CAD build for the part. Positions are in the model's coordinates, mm. Face numbers are marked on the shaded views. A direction names the side the tool comes from. Give positions to 0.01 mm unless a question says otherwise; leave off trailing zeros. Write each loop counter-clockwise with the first axis right and the second up, starting at its lowest first coordinate (ties: lowest second). Pieces come first, ordered by that corner, then holes. Notation, with made-up numbers: (62.5, 77.25) - (70.5, 77.25) arc R23 cw to (70.5, 107.25) - close; hole circle Ø6 at (-14, 75.5). An arc over 180 degrees is marked (long way). Answer as a JSON object with one key per item and string values.
from build123d import *

# Parameters (mm, degrees)
SKETCH1_R               = 15.5
SKETCH1_R_2             = 13.5
BOSS_EXTRUDE1_DEPTH     = 18
SKETCH1_3_R             = 13.5
BOSS_EXTRUDE2_DEPTH     = 3
SKETCH2_R               = 1.65
SKETCH2_R_2             = 5.2
CUT_EXTRUDE4_DEPTH      = 41
CUT_EXTRUDE5_DEPTH      = 2
CUT_EXTRUDE6_DEPTH      = 20
CUT_EXTRUDE6_DEPTH_BACK = 16
BOSS_EXTRUDE3_START     = 9
SKETCH5_R               = 15.5
SKETCH5_R_2             = 13.5
BOSS_EXTRUDE3_DEPTH     = 9


with BuildPart() as part:
    # Sketch1 → Boss-Extrude1 (new body)
    with BuildSketch(Plane(origin=(0, 0, 0), x_dir=(1, 0, 0), z_dir=(0, 1, 0))):
        with Locations(Location((0, 0, 0), (0, 0, 270))):
            Circle(SKETCH1_R)
        with Locations(Location((0, 0, 0), (0, 0, 270))):
            Circle(SKETCH1_R_2, mode=Mode.SUBTRACT)
    extrude(amount=BOSS_EXTRUDE1_DEPTH)

    # Sketch1_3 → Boss-Extrude2 (add)
    with BuildSketch(Plane(origin=(0, 0, 0), x_dir=(1, 0, 0), z_dir=(0, 1, 0))):
        with Locations(Location((0, 0, 0), (0, 0, 270))):
            Circle(SKETCH1_3_R)
    extrude(amount=BOSS_EXTRUDE2_DEPTH)

    # Sketch2 → Cut-Extrude4 (cut)
    with BuildSketch(Plane(origin=(0, 3, 0), x_dir=(1, 0, 0), z_dir=(0, 1, 0))):
        with Locations(Location((-5.654252066, 5.659455236, 0), (0, 0, 270))):
            Circle(SKETCH2_R)
        with Locations(Location((5.654252066, -5.659455236, 0), (0, 0, 270))):
            Circle(SKETCH2_R)
        with Locations(Location((5.659455236, 5.654252066, 0), (0, 0, 270))):
            Circle(SKETCH2_R)
        with Locations(Location((0, 0, 0), (0, 0, 270))):
            Circle(SKETCH2_R_2)
        with Locations(Location((-5.659455236, -5.654252066, 0), (0, 0, 270))):
            Circle(SKETCH2_R)
    extrude(amount=-CUT_EXTRUDE4_DEPTH, mode=Mode.SUBTRACT)

    # Sketch3 → Cut-Extrude5 (cut)
    with BuildSketch(Plane(origin=(0, 3, 0), x_dir=(1, 0, 0), z_dir=(0, 1, 0))):
        Polygon((-7.834437444, 3.350748878), (-4.744946398, 2.617006135), (-2.56476102, 4.925712494), (-3.474066688, 7.968161595), (-6.563557734, 8.701904338), (-8.743743112, 6.393197979), align=None)
        Polygon((3.350748878, 7.834437444), (2.617006135, 4.744946398), (4.925712494, 2.56476102), (7.968161595, 3.474066688), (8.701904338, 6.563557734), (6.393197979, 8.743743112), align=None)
        Polygon((7.834437444, -3.350748878), (4.744946398, -2.617006135), (2.56476102, -4.925712494), (3.474066688, -7.968161595), (6.563557734, -8.701904338), (8.743743112, -6.393197979), align=None)
        Polygon((-3.350748878, -7.834437444), (-2.617006135, -4.744946398), (-4.925712494, -2.56476102), (-7.968161595, -3.474066688), (-8.701904338, -6.563557734), (-6.393197979, -8.743743112), align=None)
    extrude(amount=-CUT_EXTRUDE5_DEPTH, mode=Mode.SUBTRACT)

    # Sketch4 → Cut-Extrude6 (cut, two sides: drawn at the far end of the back side and taken through both)
    with BuildSketch(Plane.XY.offset(-CUT_EXTRUDE6_DEPTH_BACK)):
        with BuildLine():
            Line((4.848949803, 5.4), (-4.848949803, 5.4))
            ThreePointArc((-4.848949803, 5.4), (-6.448949803, 7), (-4.848949803, 8.6))
            Line((-4.848949803, 8.6), (4.848949803, 8.6))
            ThreePointArc((4.848949803, 8.6), (6.448949803, 7), (4.848949803, 5.4))
        make_face()
    extrude(amount=CUT_EXTRUDE6_DEPTH + CUT_EXTRUDE6_DEPTH_BACK, mode=Mode.SUBTRACT)

    # Sketch5 → Boss-Extrude3 (add)
    with BuildSketch(Plane.XZ.offset(BOSS_EXTRUDE3_START)):
        with Locations(Location((0, 0, 0), (0, 0, 270))):
            Circle(SKETCH5_R)
        with Locations(Location((0, 0, 0), (0, 0, 90))):
            Circle(SKETCH5_R_2, mode=Mode.SUBTRACT)
    extrude(amount=-BOSS_EXTRUDE3_DEPTH)


solid = part.part
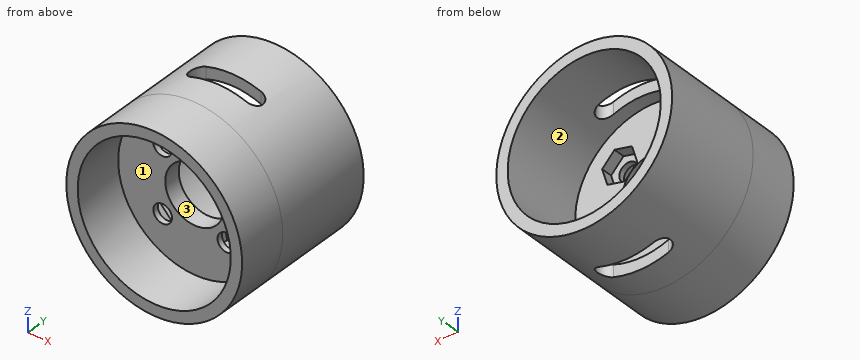
Item 1: Probe line 1 (X direction, y = -4, z = 0); line 2 (Z direction, x = 0.5, y = 16.25); line 3 (X direction, y = 2.25, z = 7). List the from-to ranges inside material, lowest first. Write a range as from..to.
Entries:
{"line 1": "-15.5..-13.5, 13.5..15.5", "line 2": "-15.49..-13.49, 13.49..15.49", "line 3": "-13.83..-8.24, -3.15..3.18, 8.17..13.83"}
Item 2: Which spindle directions (+Z, -Z, +X, -X, +Y, -Y) get a long thin tool onto all of the face, cutting with end or side? Do the marked faces 1, 2 and 3. Say none if no direction does.
Entries:
{"face 1": "-Y", "face 2": "+Y", "face 3": "+Y, -Y"}
Item 3: Cut at A-A (z = 0). Give the cut face in (x, y).
Entries:
{"outline": "(-15.5, -9) - (-13.5, -9) - (-13.5, 0) - (-5.2, 0) - (-5.2, 3) - (-13.5, 3) - (-13.5, 18) - (-15.5, 18) - close; (5.2, 0) - (13.5, 0) - (13.5, -9) - (15.5, -9) - (15.5, 18) - (13.5, 18) - (13.5, 3) - (5.2, 3) - close"}
Item 4: Cut at C-C (y = 7). Give the cut face in (x, z).
Entries:
{"outline": "(-6.45, -14.09) - (-6.45, -11.86) arc R13.5 cw to (-6.45, 11.86) - (-6.45, 14.09) arc R15.5 ccw to start; (6.45, -14.09) arc R15.5 ccw to (6.45, 14.09) - (6.45, 11.86) arc R13.5 cw to (6.45, -11.86) - close"}
Item 5: Cut at D-D (x = -9.5). Give the cut face in (y, z), and give its area (3 significant figures).
Entries:
{"outline": "(-9, -12.25) - (18, -12.25) - (18, -9.59) - (3, -9.59) - (3, 9.59) - (18, 9.59) - (18, 12.25) - (-9, 12.25) - (-9, 9.59) - (0, 9.59) - (0, -9.59) - (-9, -9.59) - close", "area": "201 mm2"}
Item 6: Flat gauge pins, fed straight in: P1, Ø2.5, axis at x = 5.65, z = 5.66, coming from the +Y side; P2, Ø5, axis at y = 12.5, z = -7, coming from the -X side; P3, Ø4, axis at y = 14.5, z = -12, coming from the +X side; P4, Ø12, axis at x = -11.5, y = 2.5, coming from the +Z side. Where does each tip first touch, or does it go through?
Entries:
{"P1": "through", "P2": "x = -14.83", "P3": "x = 11.84", "P4": "z = 14.49"}
Item 7: Cut at B-B (x = 0). Give the cut face in (y, z).
Entries:
{"outline": "(-9, -15.5) - (5.4, -15.5) - (5.4, -13.5) - (3, -13.5) - (3, -5.2) - (0, -5.2) - (0, -13.5) - (-9, -13.5) - close; (-9, 13.5) - (0, 13.5) - (0, 5.2) - (3, 5.2) - (3, 13.5) - (5.4, 13.5) - (5.4, 15.5) - (-9, 15.5) - close; (8.6, -15.5) - (18, -15.5) - (18, -13.5) - (8.6, -13.5) - close; (8.6, 13.5) - (18, 13.5) - (18, 15.5) - (8.6, 15.5) - close"}
